For this review, take the finished solid that the model builds, in its own axes (mm). A direction names the side the tool comes from. Round coordinates to 2 decimals unless told otherwise and drop trailing zeros. Order: outer loops, then holes, each group sorted by start corner. A loop starts at its lowest first (then second) coordinate and runs counter-clockwise, first axis right, second up. Notation, with made-up numbers: M 74,71.5 L 83,71.5 A36 ccw 83,105.5 Z; hole C 56.25,85.5 d9. An arc over 180 degrees is marked long. Answer as a JSON object with one key per item and string values.
Autodesk Inventor part; units mm, degrees
ref_plane "YZ Plane" through (0, 0, 0) normal (1, 0, 0) x (0, 1, 0)
ref_plane "XZ Plane" through (0, 0, 0) normal (0, 1, 0) x (-1, 0, 0)
ref_plane "XY Plane" through (0, 0, 0) normal (0, 0, 1) x (1, 0, 0)
sketch "Эскиз9" plane through (0, 0, 0) normal (0, 0, 1) x (1, 0, 0)
  line L0 (-15, -5) -> (-5, -5)
  line L1 (0, -5) -> (-5, -5)
  line L2 (5, -5) -> (0, -5)
  line L3 (5, -5) -> (15, -5)
  line L4 (-15, -10) -> (15, -10)
  line L5 (-15, -5) -> (-15, -10)
  line L6 (-15, -5) -> (15, -5)
  line L7 (15, -10) -> (15, -5)
  line L8 (15, -10) -> (-15, -10)
  line L9 (-15, -5) -> (-15, -10)
extrude "Выдавливание9" [suppressed]
sketch "Эскиз8" plane through (0, 0, 0) normal (0, 0, 1) x (1, 0, 0)
  line L0 (0, 5) -> (0, -5)
  line L1 (-5, 0) -> (5, 0)
  arc A0 (5, 0) -> (-5, 0) centre (0, 0) ccw
  line L2 (-5, 0) -> (-5, -5)
  line L3 (5, 0) -> (5, -5)
  line L4 (0, -5) -> (-4, -5)
  line L5 (4, -5) -> (0, -5)
  line L6 (-4, -5) -> (-4, 0)
  arc A1 (4, 0) -> (-4, 0) centre (0, 0) ccw
  line L7 (4, 0) -> (4, -5)
  line L8 (-5, -5) -> (-4, -5)
  line L9 (4, -5) -> (5, -5)
  line L10 (-15, -5) -> (-5, -5)
  line L11 (0, -5) -> (-5, -5)
  line L12 (5, -5) -> (0, -5)
  line L13 (5, -5) -> (15, -5)
  line L14 (-15, -10) -> (15, -10)
  line L15 (-15, -5) -> (-15, -10)
  line L16 (-15, -5) -> (15, -5)
  line L17 (15, -10) -> (15, -5)
  line L18 (15, -10) -> (-15, -10)
  line L19 (-15, -5) -> (-15, -10)
  dimension "d32" = 10
  dimension "d33" = 5
  dimension "d34" = 5
  dimension "d52" = 1
extrude "Выдавливание14" add sketch "Эскиз8" along normal blind 80
sketch "Эскиз10" plane through (-5, -5, 0) normal (-1, 0, 0) x (0, 0, 1)
  line L0 (0, 10) -> (80, 10)
  line L1 (0, 0) -> (80, 0)
  line L2 (0, 5) -> (80, 5)
  line L3 (7.9097, 10) -> (7.9097, 0)
  line L4 (0, 0) -> (80, 0)
  line L5 (12.9097, 0) -> (12.9097, 5)
  line L6 (7.9097, 0) -> (12.9097, 0)
  line L7 (12.9097, 5) -> (23.7841, 5)
  line L8 (23.7841, 0) -> (12.9097, 0)
  line L9 (23.7841, 5) -> (23.7841, 0)
  line L10 (7.9097, 10) -> (28.7841, 10)
  line L11 (28.7841, 0) -> (28.7841, 10)
  line L12 (28.7841, 0) -> (23.7841, 0)
  dimension "d64" = 5
  dimension "d65" = 5
extrude "Выдавливание15" cut sketch "Эскиз10" against normal blind 2 contours L0 L11 L2 L3 | L2 L5 L1 L3 | L11 L1 L9 L2
extrude "Выдавливание16" cut sketch "Эскиз8" along normal blind 80 contours A1 L1 L0 | L0 L1 A1 | L1 L7 L5 L0 | L0 L4 L6 L1
equation "\"d32\" = diametr_"
equation "\"d64\" = diametr_ruchka_"
equation "\"d65\" = diametr_ruchka_"
properties part number "lw_5_корпус"
1) Add section B-B on y = -1.25. State the section outline as (x, z) points.
Geometry check:
{"outline": "M -5,0 L -4,0 L -4,7.91 L -5,7.91 Z; M -5,12.91 L -4,12.91 L -4,23.78 L -5,23.78 Z; M -5,28.78 L -4,28.78 L -4,80 L -5,80 Z; M 4,0 L 5,0 L 5,80 L 4,80 Z"}
2) Machinability: for faces 1 (the flat face through (-5, -2, 18)), 2 (the flat face through (-4, -3, 54)), 3 (the flat face through (5, -2, 39)), which of the approach directions +Z, -Z, +X, -X, +Y, -Y give a long, thin tool a straight path to every point of the face, cutting with its end or side? Answer none if there is none.
Geometry check:
{"face 1": "+Z, -Z, -X, +Y", "face 2": "+Z, -Z", "face 3": "+Z, -Z, +X, +Y"}
3) Add section A-A on x = 0. State the section outline as (y, z) points, and give its area (3 significant figures).
Geometry check:
{"outline": "M -10,0 L -5,0 L -5,80 L -10,80 Z; M 4,0 L 5,0 L 5,80 L 4,80 Z", "area": "480 mm²"}
4) Insertion check: P1, Ø1.5, axis at y = -1.5, z = 5, coming from the +X side; P2, Ø1.1, axis at y = 3.5, z = 23.5, coming from the -X side; P3, Ø1.5, axis at y = 3, z = 50, coming from the -X side; P4, Ø1.5, axis at x = 7, y = -0.5, coming from the -Z side. Each pin has a flat end and moves straight along its axis. Give the tip position at first contact, or say it passes through.
Geometry check:
{"P1": "stops at x = 5", "P2": "stops at x = -3", "P3": "stops at x = -4.47", "P4": "passes through"}
5) For L1, parallel to X at y = -0.25, z = 53; L2, parallel to Y at x = 0, z = 21; L3, parallel to Y at x = -2.75, z = 52.5, list the stretches that pass through material, from the lowest coordinate up.
Geometry check:
{"L1": "x = -5 to -4, 4 to 5", "L2": "y = -10 to -5, 4 to 5", "L3": "y = -10 to -5, 2.9 to 4.18"}
6) Add section C-C on z = 36. State the section outline as (x, y) points.
Geometry check:
{"outline": "M -15,-10 L 15,-10 L 15,-5 L 5,-5 L 5,0 A5 ccw -5,0 L -5,-5 L -15,-5 Z; hole M -4,-5 L 4,-5 L 4,0 A4 ccw -4,0 Z"}
7) Mouldability with a two-part tool opening along Z and no side actions: class faces 4 (the flat face through (0, -6, 0)), 5 (the flat face through (-4.2, -0.6, 28.784)), 6 (the flat face through (4, -2, 39)) as +Z half, -Z half, draft (parallel to the pull), parting line (faces both ways), or undercut.
Geometry check:
{"face 4": "-Z half", "face 5": "undercut", "face 6": "draft"}
8) Add section D-D on z = 24.5. State the section outline as (x, y) points.
Geometry check:
{"outline": "M -15,-10 L 15,-10 L 15,-5 L 5,-5 L 5,0 A5 ccw -3,4 L -3,2.65 A4 cw 4,0 L 4,-5 L -15,-5 Z"}
